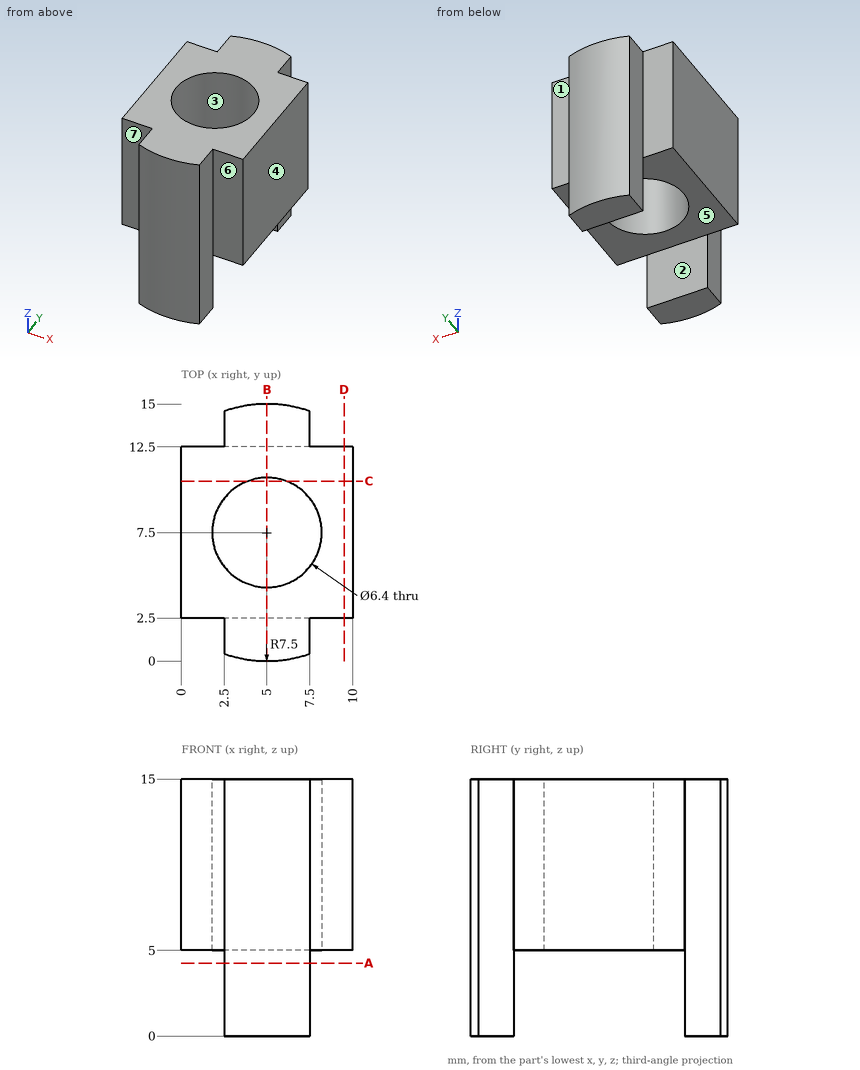
Job drawing, mm, ordinate dimensions from the low corner. One solid piece. A direction names the side the tool comes from. Coordinates: 2 decimals unless noted, no trailing zeros. Write each loop counter-clockwise with the first axis right and the second up, starting at its lowest first coordinate (ties: lowest second). Pieces come first, ordered by that corner, then holes. Notation, with made-up numbers: M 89,-26 L 99,-26 A23 ccw 99,-14 Z; hole C -1.5,83.5 d11. An arc over 180 degrees is marked long. Answer as a JSON object with one key per item and string values. Group by question number.
1) Wall check: line 1 (Y direction, x = 5, z = 11.5); line 2 (X direction, y = 5.5, z = 5.5); line 3 (Y direction, x = 3.5, z = 3). Give the ranges that are in metal, low to high. Write a range as from..to.
2) Pin check, flat tips, straight feed: pin 1 Ø0.8 at (x, z) = (9, 10) entering from +Y; pin 2 Ø0.8 at (x, z) = (9, 10.5) entering from -Y; pin 3 Ø1 at (y, z) = (13.5, 9) entering from +X. Stop position of each tip, or through.
3) Saw through at B-B (x = 5). Write the cut outline in (y, z), plus the area to 3 significant figures.
4) Saw through at A-A (z = 4.25). Write the cut outline in (x, y), plus the area to 3 significant figures.
5) Mould opens along Y. For the marked faces 1, 2, 3 and 4 say: +Y half, -Y half, draft (parallel to the pull), parting line (faces both ways), or undercut.
6) Tool access for the marked faces 5, 6 and 7: list every direction of +Z, -Z, +X, -X, +Y, -Y with a clear straight run to the whole face (end or side of a thin tool).
7) Saw through at C-C (y = 10.5). Write the cut outline in (x, z).
8) Saw through at D-D (x = 9.5). Write the cut outline in (y, z).
Values follow:
{
 "1": {"line 1": "y = 0..4.3, 10.7..15", "line 2": "x = 0..2.5, 7.5..10", "line 3": "y = 0.15..2.5, 12.5..14.85"},
 "2": {"pin 1": "stops at y = 12.5", "pin 2": "stops at y = 2.5", "pin 3": "stops at x = 7.5"},
 "3": {"outline": "M 0,0 L 2.5,0 L 2.5,5 L 4.3,5 L 4.3,15 L 0,15 Z; M 10.7,5 L 12.5,5 L 12.5,0 L 15,0 L 15,15 L 10.7,15 Z", "area": "111 mm2"},
 "4": {"outline": "M 2.5,0.43 A7.5 ccw 7.5,0.43 L 7.5,2.5 L 2.5,2.5 Z; M 2.5,12.5 L 7.5,12.5 L 7.5,14.57 A7.5 ccw 2.5,14.57 Z", "area": "23.6 mm2"},
 "5": {"face 1": "+Y half", "face 2": "undercut", "face 3": "undercut", "face 4": "draft"},
 "6": {"face 5": "-Z, +X, -X", "face 6": "+Z, -Z, +X, -Y", "face 7": "+Z, -Z, -X, -Y"},
 "7": {"outline": "M 0,5 L 3.89,5 L 3.89,15 L 0,15 Z; M 6.11,5 L 10,5 L 10,15 L 6.11,15 Z"},
 "8": {"outline": "M 2.5,5 L 12.5,5 L 12.5,15 L 2.5,15 Z"}
}
